from build123d import *

# Parameters (mm, degrees)
SKETCH2_R                = 5
BOSS_EXTRUDE1_DEPTH      = 15
BOSS_EXTRUDE2_DEPTH      = 10
BOSS_EXTRUDE2_DEPTH_BACK = 50


with BuildPart() as part:
    # Sketch2 → Boss-Extrude1 (new body)
    with BuildSketch(Plane(origin=(0, 0, 0), x_dir=(0, 0, -1), z_dir=(1, 0, 0))):
        Circle(SKETCH2_R)
    extrude(amount=-BOSS_EXTRUDE1_DEPTH)

    # Sketch3 → Boss-Extrude2 (add, two sides)
    with BuildSketch(Plane.XY) as boss_extrude2_sk:
        Polygon((-15, 0), (-15, 10), (-30, 10), (-30, -10), (-15, -10), align=None)
    extrude(amount=BOSS_EXTRUDE2_DEPTH)
    extrude(boss_extrude2_sk.sketch, amount=-BOSS_EXTRUDE2_DEPTH_BACK)


solid = part.part
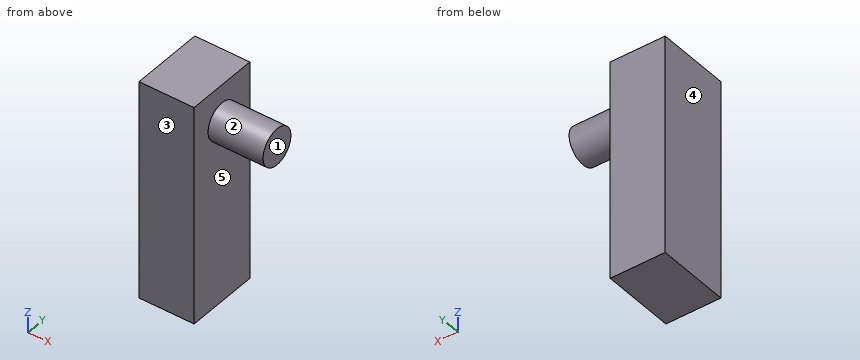
Could you check a few things on this model? Use its own coordinates, in mm. Face numbers are marked on the shaded views. A direction names the side the tool comes from. Coordinates: 2 decimals unless noted, no trailing zeros. Order: outer loops, then holes, each group sorted by start corner. A loop starts at its lowest first (then second) coordinate and runs counter-clockwise, first axis right, second up. Notation, with made-up numbers: (-7, 49) -> (9, 49) arc R18 cw to (9, 58) -> close; hole circle Ø10 at (37.25, -33). An arc over 180 degrees is marked (long way). One line per item, written item: value. Start each with the question number.
1) If I drill on L1, parallel to X at y = 6, z = -43; L2, parallel to Z at x = -4, y = 1; L3, parallel to Z at x = -7, y = -2.5, over which ranges is the centre line in solid material (lowest first)? Write a range as [from, to].
2) Imagine slicing it at C-C on y = -8.25. List the corners of the cut face in (x, z) for me.
3) Imagine slicing it at B-B on z = 0. List the corners of the cut face in (x, y) for me, plus the area to 3 significant figures.
4) I'm going to push flat-ended pins straight in: pin 1 (3 mm diameter, centred on x = -14, y = -4.5, fed in from +Z); pin 2 (3 mm diameter, centred on x = -13, y = 0, fed in from -Z); pin 3 (1 mm diameter, centred on x = -13.5, y = 6, fed in from -Z); pin 4 (5 mm diameter, centred on x = -5, y = 4.5, fed in from -Z). Where does each tip first touch, or does it pass through?
5) We'd pull the mould along X, two halves only. Please class the marked faces 3, 4 and 5: +X half, -X half, draft (parallel to the pull), parting line (faces both ways), or undercut.
6) Imagine slicing it at A-A on y = 0. List the corners of the cut face in (x, z) for me, plus the area to 3 significant figures.
7) Imagine slicing it at D-D on z = -9. List the corners of the cut face in (x, y) for me, plus the area to 3 significant figures.
8) Which directions (+Z, -Z, +X, -X, +Y, -Y) give clear straight access to the entire face, cutting with the end or side of a thin tool? Please do the marked faces 1 and 2.
Answer list:
1. L1: x = [-30, -15]
1. L2: z = [-4.9, 4.9]
1. L3: z = [-4.33, 4.33]
2. outline: (-30, -50) -> (-15, -50) -> (-15, 10) -> (-30, 10) -> close
3. outline: (-30, -10) -> (-15, -10) -> (-15, -5) -> (0, -5) -> (0, 5) -> (-15, 5) -> (-15, 10) -> (-30, 10) -> close
3. area: 450 mm2
4. pin 1: stops at z = 10
4. pin 2: stops at z = -5
4. pin 3: passes through
4. pin 4: stops at z = -4.58
5. face 3: draft
5. face 4: -X half
5. face 5: +X half
6. outline: (-30, -50) -> (-15, -50) -> (-15, -5) -> (0, -5) -> (0, 5) -> (-15, 5) -> (-15, 10) -> (-30, 10) -> close
6. area: 1,050 mm2
7. outline: (-30, -10) -> (-15, -10) -> (-15, 10) -> (-30, 10) -> close
7. area: 300 mm2
8. face 1: +Z, -Z, +X, +Y, -Y
8. face 2: +X
